Geometry: final body of the model. Coordinates: model frame, mm. Face numbers are marked on the shaded views. A direction names the side the tool comes from. Give positions to 0.01 mm unless a question says otherwise; leave off trailing zeros. Order: outer loops, then holes, each group sorted by start corner. A loop starts at its lowest first (then second) coordinate and runs counter-clockwise, first axis right, second up. Notation, with made-up numbers: (40, -17) - (87, -17) arc R13 ccw to (87, 4) - close; hole circle Ø4 at (1.5, 89.5). An arc over 180 degrees is marked (long way). One line per item, written item: value.
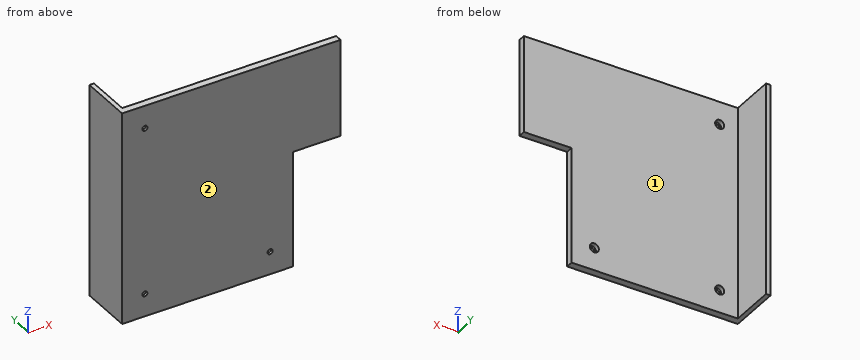
```python
from build123d import *

# Parameters (mm, degrees)
SKETCH1_W                      = 192.4
SKETCH1_H                      = 187.4
BOSS_EXTRUDE1_DEPTH            = 6.35
BOSS_EXTRUDE2_DEPTH            = 40
CUT_EXTRUDE1_REACH             = 142.122
SKETCH4_W                      = 42
SKETCH4_H                      = 102
CBORE_FOR_M4_SHCS1_D           = 4.5
CBORE_FOR_M4_SHCS1_CBORE_D     = 8
CBORE_FOR_M4_SHCS1_CBORE_DEPTH = 4


with BuildPart() as part:
    # Sketch1 → Boss-Extrude1 (new body)
    with BuildSketch(Plane(origin=(0, 0, 0), x_dir=(1, 0, 0), z_dir=(0, 1, 0))):
        Rectangle(SKETCH1_W, SKETCH1_H)
    extrude(amount=BOSS_EXTRUDE1_DEPTH)

    # Sketch2 → Boss-Extrude2 (add)
    with BuildSketch(Plane(origin=(0, 6.35, 0), x_dir=(1, 0, 0), z_dir=(0, 1, 0))):
        Polygon((-92.2, 89.7), (-92.2, -89.7), (-92.2, -93.7), (-96.2, -93.7), (-96.2, 93.7), (-92.2, 93.7), align=None)
    extrude(amount=BOSS_EXTRUDE2_DEPTH)

    # Sketch4 → Cut-Extrude1 (cut, up to next)
    with BuildSketch(Plane(origin=(0, 6.35, 0), x_dir=(1, 0, 0), z_dir=(0, 1, 0)), mode=Mode.PRIVATE) as cut_extrude1_sk1:
        with Locations((75.2, 42.7)):
            Rectangle(SKETCH4_W, SKETCH4_H)
    cut_extrude1_tool1 = extrude(cut_extrude1_sk1.sketch, amount=-CUT_EXTRUDE1_REACH, mode=Mode.PRIVATE) & part.part
    add(cut_extrude1_tool1.solids().sort_by_distance((75.2, 6.35, -42.7))[0], mode=Mode.SUBTRACT)

    # CBORE for M4 SHCS1 (through all)
    with Locations(Plane(origin=(0, 6.35, 0), x_dir=(1, 0, 0), z_dir=(0, 1, 0))):
        with Locations((34.2, 73.7), (-76.2, 73.7), (-76.2, -73.7)):
            CounterBoreHole(CBORE_FOR_M4_SHCS1_D / 2, CBORE_FOR_M4_SHCS1_CBORE_D / 2, CBORE_FOR_M4_SHCS1_CBORE_DEPTH)


solid = part.part
```
1) Section C-C, the plane x = -76.2. Return loops of the section in (y, z), then the cut area to 3 significant figures.
Answers below:
outline: (0, -93.7) - (6.35, -93.7) - (6.35, -77.7) - (2.35, -77.7) - (2.35, -75.95) - (0, -75.95) - close; (0, -71.45) - (2.35, -71.45) - (2.35, -69.7) - (6.35, -69.7) - (6.35, 69.7) - (2.35, 69.7) - (2.35, 71.45) - (0, 71.45) - close; (0, 75.95) - (2.35, 75.95) - (2.35, 77.7) - (6.35, 77.7) - (6.35, 93.7) - (0, 93.7) - close
area: 1,100 mm^2
2) Section D-D, the plane z = 31.5. Return loops of the section in (x, y), then the cut area to 3 significant figures.
Answers below:
outline: (-96.2, 0) - (96.2, 0) - (96.2, 6.35) - (-92.2, 6.35) - (-92.2, 46.35) - (-96.2, 46.35) - close
area: 1,380 mm^2
3) First-contact query: pin 1 (4 mm diameter, centred on x = -78, z = 75.5, fed in from +Y); pin 2 (4 mm diameter, centred on y = 37, z = -19.5, fed in from +X); pin 3 (7 mm diameter, centred on x = -76.2, z = -73.7, fed in from +Y); pin 4 (2.5 mm diameter, centred on x = 34.2, z = -73.7, fed in from +Y). Flat tips, straight axial feed; report the tip coordinate or a pass-through.
Answers below:
pin 1: y = 6.35
pin 2: x = -92.2
pin 3: y = 2.35
pin 4: through
4) Set-up query: the marked faces 1 and 2. Return all of +Z, -Z, +X, -X, +Y, -Y with unobstructed straight access to the full face (end or side cutting, diameter ignored); none if empty.
Answers below:
face 1: +Z, -Z, +X, +Y
face 2: +Z, -Z, +X, -X, -Y
5) Section A-A, the plane z = 73.7. Return loops of the section in (x, y), then the cut area to 3 significant figures.
Answers below:
outline: (-96.2, 0) - (-78.45, 0) - (-78.45, 2.35) - (-80.2, 2.35) - (-80.2, 6.35) - (-92.2, 6.35) - (-92.2, 46.35) - (-96.2, 46.35) - close; (-73.95, 0) - (96.2, 0) - (96.2, 6.35) - (-72.2, 6.35) - (-72.2, 2.35) - (-73.95, 2.35) - close
area: 1,340 mm^2
6) Section B-B, the plane x = 34.2. Return loops of the section in (y, z), then the cut area to 3 significant figures.
Answers below:
outline: (0, -93.7) - (6.35, -93.7) - (6.35, -77.7) - (2.35, -77.7) - (2.35, -75.95) - (0, -75.95) - close; (0, -71.45) - (2.35, -71.45) - (2.35, -69.7) - (6.35, -69.7) - (6.35, 93.7) - (0, 93.7) - close
area: 1,150 mm^2
7) Material intervals for line 1 along Z through (x, y) = (-76.2, 4.45); line 2 along X through (y, z) = (1.05, -73.7); line 3 along Z through (x, y) = (-76.2, 0.7), sorted ascending.
Answers below:
line 1: -93.7 to -77.7, -69.7 to 69.7, 77.7 to 93.7
line 2: -96.2 to -78.45, -73.95 to 31.95, 36.45 to 54.2
line 3: -93.7 to -75.95, -71.45 to 71.45, 75.95 to 93.7
